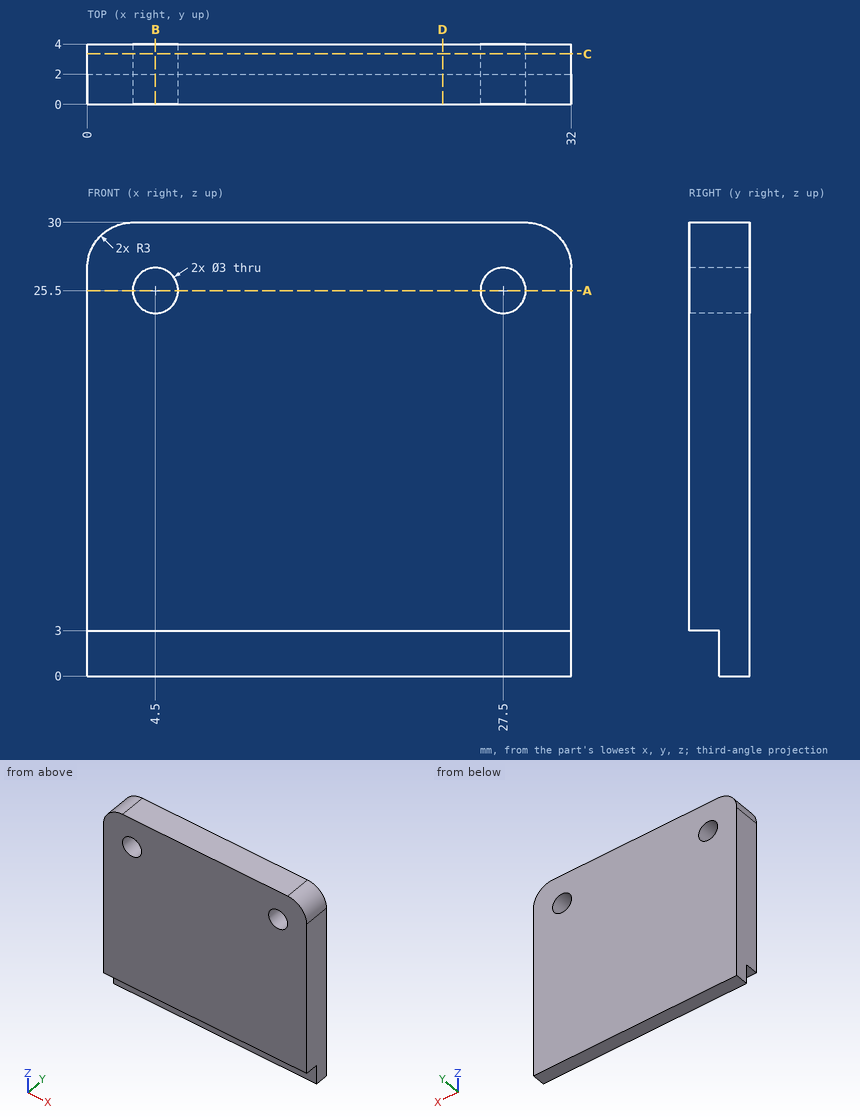
Design review of the part shown in the three views and the two pictorial views. Dimensions are in mm from the part's minimum x, y and z. Coordinates: 2 decimals unless noted, no trailing zeros. Order: outer loops, then holes, each group sorted by start corner. A loop starts at its lowest first (then second) coordinate and runs counter-clockwise, first axis right, second up. Notation, with made-up numbers: (-32.5, 2) -> (4.5, 2) arc R30 ccw to (4.5, 40) -> close; hole circle Ø1 at (55.5, -12). An arc over 180 degrees is marked (long way). Use one line per item in the form item = value. Start each with the question number.
(1) Add section D-D on x = 23.5. State the section outline as (y, z) points.
(2) For probe 1 along Z at (x, y) = (27.5, 1.75); probe 2 along Z at (x, y) = (27.5, 2.85); probe 3 along Z at (x, y) = (18, 0.65), list the stretches that pass through material, from the lowest coordinate up.
(3) Add section B-B on x = 4.5. State the section outline as (y, z) points.
(4) Add section A-A on z = 25.5. State the section outline as (x, y) points, plus the area to 3 significant figures.
(5) Insertion check: pin 1 (1 mm diameter, centred on y = 3, z = 6, fed in from -X); pin 2 (1.5 mm diameter, centred on x = 6, y = 0.5, fed in from -Z); pin 3 (2.5 mm diameter, centred on x = 23, z = 1, fed in from -Y). Each pin has a flat end and moves straight along its axis. Give the tip position at first contact, or say it passes through.
(6) Add section C-C on y = 3.35. State the section outline as (x, z) points.
Answer block:
q1.outline = (0, 3) -> (2, 3) -> (2, 0) -> (4, 0) -> (4, 30) -> (0, 30) -> close
q2.probe_1 = 3 to 24, 27 to 30
q2.probe_2 = 0 to 24, 27 to 30
q2.probe_3 = 3 to 30
q3.outline = (0, 3) -> (2, 3) -> (2, 0) -> (4, 0) -> (4, 24) -> (0, 24) -> close; (0, 27) -> (4, 27) -> (4, 30) -> (0, 30) -> close
q4.outline = (0, 0) -> (3, 0) -> (3, 4) -> (0, 4) -> close; (6, 0) -> (26, 0) -> (26, 4) -> (6, 4) -> close; (29, 0) -> (32, 0) -> (32, 4) -> (29, 4) -> close
q4.area = 104 mm²
q5.pin_1 = 0
q5.pin_2 = 3
q5.pin_3 = 2
q6.outline = (0, 0) -> (32, 0) -> (32, 27) arc R3 ccw to (29, 30) -> (3, 30) arc R3 ccw to (0, 27) -> close; hole circle Ø3 at (4.5, 25.5); hole circle Ø3 at (27.5, 25.5)
